Model file for the job. Use its own axes, mm. A direction names the side the tool comes from. Round coordinates to 2 decimals unless told otherwise and drop trailing zeros. Loops run counter-clockwise (first coordinate to the right, second up) from the corner with the lowest first, then second, coordinate; pieces in that order, holes last. Notation, with made-up numbers: (-11.5, 5.5) -> (-7.5, 5.5) arc R18 cw to (-7.5, 17.5) -> close; hole circle Ø4 at (10, 67). An arc over 180 degrees is marked (long way). Use a Markdown table: item, result.
from build123d import *

# Parameters (mm, degrees)
BOSS_EXTRUDE1_DEPTH = 40
CUT_EXTRUDE1_DEPTH  = 88
SHELL1_START        = -88.5
SHELL1_DEPTH        = 80
BOSS_EXTRUDE2_REACH = 116.334
SKETCH3_R           = 4.175
SKETCH3_3_R         = 4.175
BOSS_EXTRUDE3_DEPTH = 40
SKETCH4_R           = 1.575
CUT_EXTRUDE2_DEPTH  = 40
SKETCH4_3_R         = 3.15
SKETCH4_3_R_2       = 1.575
CUT_EXTRUDE3_DEPTH  = 38.5
SKETCH5_R           = 4.675
SKETCH5_R_2         = 2.175
BOSS_EXTRUDE4_DEPTH = 7.5
SKETCH6_W           = 34.1
SKETCH6_H           = 18.9
CUT_EXTRUDE4_DEPTH  = 4
CHAMFER1_SIZE       = 4
SKETCH8_R           = 2.65
CUT_EXTRUDE5_DEPTH  = 4
SKETCH9_R           = 1.4
BOSS_EXTRUDE7_DEPTH = 7.399


# Read off the part's stored shape, not the designer's step: Shell1
with BuildPart() as part:
    # Sketch1 → Boss-Extrude1 (new body)
    with BuildSketch(Plane.XY):
        with BuildLine():
            Line((-4.5, 54), (-88.5, 54))
            ThreePointArc((-88.5, 54), (-91.328427125, 52.828427125), (-92.5, 50))
            Line((-92.5, 50), (-92.5, -50))
            ThreePointArc((-92.5, -50), (-91.328427125, -52.828427125), (-88.5, -54))
            Line((-88.5, -54), (-4.5, -54))
            Line((-4.5, -54), (-4.5, 54))
        make_face()
    extrude(amount=BOSS_EXTRUDE1_DEPTH)

    # Sketch2 → Cut-Extrude1 (cut)
    with BuildSketch(Plane.ZY.offset(92.5)):
        Polygon((6.4, -50), (40, -50), (40, 6), align=None)
        Polygon((4, -54), (40, -54), (40, -50), (6.4, -50), align=None)
    extrude(amount=-CUT_EXTRUDE1_DEPTH, mode=Mode.SUBTRACT)

    # Shell1 outline → Shell1 (cut)
    with BuildSketch(Plane.YZ.offset(SHELL1_START)):
        Polygon((50, 0), (50, 36), (7.10793586, 36), (-50, 1.735238484), (-50, 0), align=None)
    extrude(amount=SHELL1_DEPTH, mode=Mode.SUBTRACT)

    # Boss-Extrude2: up to this plane
    boss_extrude2_end = Plane(origin=(65.471422738, -14.000840508, 23.33473418), z_dir=(0, 0.5144957554275265, -0.8574929257125443))
    # Sketch3 → Boss-Extrude2 (add, up to the surface)
    with BuildSketch(Plane.XY, mode=Mode.PRIVATE) as boss_extrude2_sk1:
        with Locations((-86.962042751, -48.462042751)):
            Circle(SKETCH3_R)
    boss_extrude2_tool1 = split(extrude(boss_extrude2_sk1.sketch, amount=BOSS_EXTRUDE2_REACH, mode=Mode.PRIVATE), bisect_by=boss_extrude2_end, keep=Keep.BOTH, mode=Mode.PRIVATE)
    add(boss_extrude2_tool1.solids().sort_by_distance((-86.962043, -48.462043, 0))[0])
    # Sketch3 → Boss-Extrude2 (add, up to the surface)
    with BuildSketch(Plane.XY, mode=Mode.PRIVATE) as boss_extrude2_sk2:
        with Locations((-10.037957249, -48.462042751)):
            Circle(SKETCH3_R)
    boss_extrude2_tool2 = split(extrude(boss_extrude2_sk2.sketch, amount=BOSS_EXTRUDE2_REACH, mode=Mode.PRIVATE), bisect_by=boss_extrude2_end, keep=Keep.BOTH, mode=Mode.PRIVATE)
    add(boss_extrude2_tool2.solids().sort_by_distance((-10.037957, -48.462043, 0))[0])

    # Sketch3<3> → Boss-Extrude3 (add)
    with BuildSketch(Plane.XY):
        with Locations((-86.962042751, 48.462042751)):
            Circle(SKETCH3_3_R)
        with Locations((-10.037957249, 48.462042751)):
            Circle(SKETCH3_3_R)
    extrude(amount=BOSS_EXTRUDE3_DEPTH)

    # Sketch4 → Cut-Extrude2 (cut)
    with BuildSketch(Plane.XY.offset(40)):
        with Locations((-86.962042751, 48.462042751)):
            Circle(SKETCH4_R)
        with Locations((-10.037957249, 48.462042751)):
            Circle(SKETCH4_R)
        with Locations(Location((-10.037957249, -48.462042751, 0), (0, 0, 90))):
            Circle(SKETCH4_R)
        with Locations(Location((-86.962042751, -48.462042751, 0), (0, 0, 90))):
            Circle(SKETCH4_R)
    extrude(amount=-CUT_EXTRUDE2_DEPTH, mode=Mode.SUBTRACT)

    # Sketch4<3> → Cut-Extrude3 (cut)
    # profile 1 of 4: a face of its own
    with BuildSketch(Plane.XY.offset(40)):
        with Locations((-86.962042751, 48.462042751)):
            Circle(SKETCH4_3_R)
        with Locations(Location((-86.962042751, 48.462042751, 0), (0, 0, 180))):
            Circle(SKETCH4_3_R_2, mode=Mode.SUBTRACT)
    # profile 2 of 4: a face of its own
    with BuildSketch(Plane.XY.offset(40)):
        with Locations((-10.037957249, 48.462042751)):
            Circle(SKETCH4_3_R)
        with Locations(Location((-10.037957249, 48.462042751, 0), (0, 0, 180))):
            Circle(SKETCH4_3_R_2, mode=Mode.SUBTRACT)
    # profile 3 of 4: a face of its own
    with BuildSketch(Plane.XY.offset(40)):
        with Locations(Location((-10.037957249, -48.462042751, 0), (0, 0, 90))):
            Circle(SKETCH4_3_R)
        with Locations(Location((-10.037957249, -48.462042751, 0), (0, 0, 180))):
            Circle(SKETCH4_3_R_2, mode=Mode.SUBTRACT)
    # profile 4 of 4: a face of its own
    with BuildSketch(Plane.XY.offset(40)):
        with Locations(Location((-86.962042751, -48.462042751, 0), (0, 0, 90))):
            Circle(SKETCH4_3_R)
        with Locations(Location((-86.962042751, -48.462042751, 0), (0, 0, 180))):
            Circle(SKETCH4_3_R_2, mode=Mode.SUBTRACT)
    extrude(amount=-CUT_EXTRUDE3_DEPTH, mode=Mode.SUBTRACT)

    # Sketch5 → Boss-Extrude4 (add)
    # profile 1 of 4: a face of its own
    with BuildSketch(Plane(origin=(0, -14.000840508, 23.33473418), x_dir=(-1, 0, 0), z_dir=(0, 0.5144957554275266, -0.8574929257125442))):
        with Locations(Location((79, -30.671229776, 0), (0, 0, 90))):
            Circle(SKETCH5_R)
        with Locations(Location((79, -30.671229776, 0), (0, 0, 90))):
            Circle(SKETCH5_R_2, mode=Mode.SUBTRACT)
    # profile 2 of 4: a face of its own
    with BuildSketch(Plane(origin=(0, -14.000840508, 23.33473418), x_dir=(-1, 0, 0), z_dir=(0, 0.5144957554275266, -0.8574929257125442))):
        with Locations(Location((18, -30.671229776, 0), (0, 0, 90))):
            Circle(SKETCH5_R)
        with Locations(Location((18, -30.671229776, 0), (0, 0, 90))):
            Circle(SKETCH5_R_2, mode=Mode.SUBTRACT)
    # profile 3 of 4: a face of its own
    with BuildSketch(Plane(origin=(0, -14.000840508, 23.33473418), x_dir=(-1, 0, 0), z_dir=(0, 0.5144957554275266, -0.8574929257125442))):
        with Locations(Location((79, 14.328770224, 0), (0, 0, 90))):
            Circle(SKETCH5_R)
        with Locations(Location((79, 14.328770224, 0), (0, 0, 90))):
            Circle(SKETCH5_R_2, mode=Mode.SUBTRACT)
    # profile 4 of 4: a face of its own
    with BuildSketch(Plane(origin=(0, -14.000840508, 23.33473418), x_dir=(-1, 0, 0), z_dir=(0, 0.5144957554275266, -0.8574929257125442))):
        with Locations(Location((18, 14.328770224, 0), (0, 0, 90))):
            Circle(SKETCH5_R)
        with Locations(Location((18, 14.328770224, 0), (0, 0, 90))):
            Circle(SKETCH5_R_2, mode=Mode.SUBTRACT)
    extrude(amount=BOSS_EXTRUDE4_DEPTH)

    # Sketch6 → Cut-Extrude4 (cut)
    with BuildSketch(Plane(origin=(0, -14.000840508, 23.33473418), x_dir=(-1, 0, 0), z_dir=(0, 0.5144957554275266, -0.8574929257125442))):
        with Locations((48.5, -0.994885818)):
            Rectangle(SKETCH6_W, SKETCH6_H)
    extrude(amount=-CUT_EXTRUDE4_DEPTH, mode=Mode.SUBTRACT)

    # Chamfer1
    chamfer1_edges = [part.edges().sort_by_distance(p)[0] for p in [
        (-48.5, -25.015239228, 21.390856463),
        (-31.45, -16.91193108, 26.252841352),
        (-48.5, -8.808622932, 31.114826241),
        (-65.55, -16.91193108, 26.252841352),
    ]]
    chamfer(chamfer1_edges, length=CHAMFER1_SIZE - 0.0001)  # a hair under: the kernel refuses the full size

    # Sketch8 → Cut-Extrude5 (cut)
    with BuildSketch(Plane(origin=(0, -16.058823529, 26.764705882), x_dir=(1, 0, 0), z_dir=(0, -0.5144957554275266, 0.8574929257125442))):
        with Locations(Location((-47.45, -26.521229776, 0), (0, 0, 270))):
            Circle(SKETCH8_R)
        with Locations(Location((-37.95, -26.421229776, 0), (0, 0, 270))):
            Circle(SKETCH8_R)
        with Locations(Location((-28.55, -26.421229776, 0), (0, 0, 270))):
            Circle(SKETCH8_R)
    extrude(amount=-CUT_EXTRUDE5_DEPTH, mode=Mode.SUBTRACT)

    # Sketch9 → Boss-Extrude7 (add)
    with BuildSketch(Plane(origin=(0, -14.000840508, 23.33473418), x_dir=(-1, 0, 0), z_dir=(0, 0.5144957554275266, -0.8574929257125442))):
        with Locations(Location((63, -16.344885818, 0), (0, 0, 270))):
            Circle(SKETCH9_R)
        with Locations(Location((34, -16.344885818, 0), (0, 0, 270))):
            Circle(SKETCH9_R)
        with Locations(Location((34, 10.655114182, 0), (0, 0, 270))):
            Circle(SKETCH9_R)
        with Locations(Location((63, 10.655114182, 0), (0, 0, 270))):
            Circle(SKETCH9_R)
    extrude(amount=BOSS_EXTRUDE7_DEPTH)


solid = part.part
Q1. Pull direction Z, two halves, no side cores. Call faces 1 (the face through (-79.03, -1.69, 30.72)), 2 (the face through (-85.565, -47.735, 0.761)), 3 (the face through (-34.02, -24.193, 8.591)), 4 (the face through (-67.522, -16.03, 24.417)): released by +Z, released by -Z, zero draft, split by the parting line, or undercut.
Results list:
| item | result |
|---|---|
| face 1 | undercut |
| face 2 | zero draft |
| face 3 | released by -Z |
| face 4 | released by +Z |
Q2. Band-saw the part on A-A, the plane y = 18. Give the cut face in (x, z), plus the area to 3 significant figures.
Results list:
| item | result |
|---|---|
| outline | (-92.5, 0) -> (-88.5, 0) -> (-88.5, 36) -> (-8.5, 36) -> (-8.5, 0) -> (-4.5, 0) -> (-4.5, 40) -> (-92.5, 40) -> close |
| area | 640 mm² |
Q3. Band-saw the part on B-B, the plane x = -30. Give the cut face in (y, z), plus the area to 3 significant figures.
Results list:
| item | result |
|---|---|
| outline | (-54, 0) -> (-50, 0) -> (-50, 1.74) -> (-38.56, 8.6) -> (-40.62, 12.03) -> (-54, 4) -> close; (-36.81, 14.31) -> (-34.75, 10.88) -> (7.11, 36) -> (50, 36) -> (50, 0) -> (54, 0) -> (54, 40) -> (6, 40) -> (-5.38, 33.17) -> (-6.25, 29.67) -> (-24.95, 18.46) -> (-28.45, 19.33) -> close |
| area | 539 mm² |
Q4. Tool access for faces 5 (the face through (-46, 54, 20)), 6 (the face through (-88.5, 9, 14)), 7 (the face through (-85.509, 45.667, 21.02)): list every direction of +Z, -Z, +X, -X, +Y, -Y with a clear straight run to the whole face (end or side of a thin tool).
Results list:
| item | result |
|---|---|
| face 5 | +Z, -Z, +X, -X, +Y |
| face 6 | -Z |
| face 7 | +Z |
Q5. Drill centre lines: L1, parallel to X at y = 24, z = 32.5; L2, parallel to X at y = -38.5, z = 4.5; L3, parallel to X at y = 4, z = 27.5. Where is each one in solid material? Low to high. Write a range as from..to.
Results list:
| item | result |
|---|---|
| L1 | x = -92.5..-88.5, -8.5..-4.5 |
| L2 | x = -92.5..-88.5, -83.67..-81.17, -76.83..-74.33, -22.67..-20.17, -15.83..-13.33, -8.5..-4.5 |
| L3 | x = -92.5..-88.5, -82.36..-75.64, -21.36..-14.64, -8.5..-4.5 |
Q6. Flat gauge pins, fed straight in: pin 1 (1 mm diameter, centred on x = -62, z = 23.5, fed in from -Y); pin 2 (5 mm diameter, centred on x = -86.96, y = -48.46, fed in from -Z); pin 3 (4 mm diameter, centred on x = -69.5, y = 1.5, fed in from -Z). Where does each tip first touch, or does it go through?
Results list:
| item | result |
|---|---|
| pin 1 | stops at y = -3.33 |
| pin 2 | stops at z = 0 |
| pin 3 | stops at z = 31.44 |
